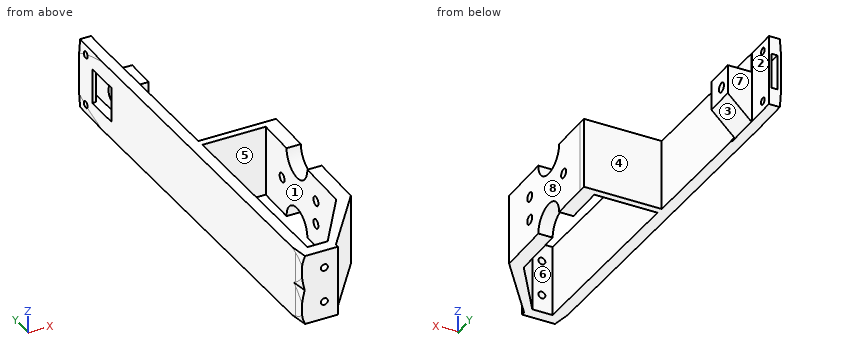
```python
from build123d import *

# Parameters (mm, degrees)
EXTRUDE1_DEPTH                 = 30
EXTRUDE2_DEPTH                 = 30
SKETCH4_R                      = 8.288803623
EXTRUDE4_DEPTH                 = 30
SKETCH5_R                      = 1.95
EXTRUDE5_DEPTH                 = 20
SKETCH6_R                      = 1.95
EXTRUDE6_DEPTH                 = 20
SKETCH9_R                      = 1.45
EXTRUDE9_DEPTH                 = 20
EXTRUDE12_DEPTH                = 171
EXTRUDE15_START                = -4
EXTRUDE15_DEPTH                = 14
SKETCH17_W                     = 15
SKETCH17_H                     = 14.5
EXTRUDE17_DEPTH                = 4
SKETCH18_W                     = 2.5
SKETCH18_H                     = 15
EXTRUDE18_DEPTH                = 10
SKETCH19_W                     = 22
SKETCH19_H                     = 13
EXTRUDE19_DEPTH                = 10
SKETCH20_R                     = 4
EXTRUDE20_DEPTH                = 8.5
SKETCH21_R                     = 2
EXTRUDE21_DEPTH                = 9
EXTRUDE22_DEPTH                = 15
F_2_9_2_9_DIAMETER_HOLE1_D     = 2.9
F_2_9_2_9_DIAMETER_HOLE1_DEPTH = 10
EXTRUDE23_DEPTH                = 32


with BuildPart() as part:
    # Sketch1 → Extrude1 (new body)
    with BuildSketch(Plane.XY):
        Polygon((-0.863115633, -23.253389327), (14.136884367, -23.253389327), (14.136884367, -21.7046417), (34.636884367, 5.336278221), (34.636884367, 61.746610673), (28.636884367, 61.746610673), (28.636884367, 5.55848015), (12.519738096, -18.253389327), (-0.863115633, -18.253389327), align=None)
    extrude(amount=EXTRUDE1_DEPTH)

    # Sketch2 → Extrude2 (add)
    with BuildSketch(Plane.XY):
        Polygon((-0.863115633, -18.253389327), (-4.863115633, 146.746610673), (-0.063115633, 146.746610673), (0.136884367, 146.746610673), (0.136884367, 138.496610673), (1.925187517, 64.729105762), (34.532746461, 64.729105762), (34.636884367, 61.746610673), (28.636884367, 61.746610673), (2.118981118, 61.746610673), (4.058375057, -18.253389327), align=None)
    extrude(amount=EXTRUDE2_DEPTH)

    # Sketch4 → Extrude4 (cut)
    with BuildSketch(Plane(origin=(34.636884367, 0, 0), x_dir=(0, 0, -1), z_dir=(1, 0, 0))):
        with Locations((0, 36.886010892)):
            Circle(SKETCH4_R)
        with Locations((-30, 36.886010892)):
            Circle(SKETCH4_R)
    extrude(amount=-EXTRUDE4_DEPTH, mode=Mode.SUBTRACT)

    # Sketch5 → Extrude5 (cut)
    with BuildSketch(Plane(origin=(34.636884367, 0, 0), x_dir=(0, 0, -1), z_dir=(1, 0, 0))):
        with Locations((-20, 21.746610673)):
            Circle(SKETCH5_R)
        with Locations((-10, 21.746610673)):
            Circle(SKETCH5_R)
    extrude(amount=-EXTRUDE5_DEPTH, mode=Mode.SUBTRACT)

    # Sketch6 → Extrude6 (cut)
    with BuildSketch(Plane(origin=(34.636884367, 0, 0), x_dir=(0, 0, -1), z_dir=(1, 0, 0))):
        with Locations((-15, 48.746610673)):
            Circle(SKETCH6_R)
    extrude(amount=-EXTRUDE6_DEPTH, mode=Mode.SUBTRACT)

    # Sketch9 → Extrude9 (cut)
    with BuildSketch(Plane.XZ.offset(23.253389327)):
        with Locations((8.519738096, 7.5)):
            Circle(SKETCH9_R)
        with Locations((8.519738096, 22.5)):
            Circle(SKETCH9_R)
    extrude(amount=-EXTRUDE9_DEPTH, mode=Mode.SUBTRACT)

    # Sketch14 → Extrude12 (cut, through all)
    with BuildSketch(Plane(origin=(0, 146.746610673, 0), x_dir=(-1, 0, 0), z_dir=(0, 1, 0))):
        with BuildLine():
            Line((4.441840203, 0), (4.863115633, 0))
            Line((4.863115633, 0), (4.863115633, 6.019259174))
            add(Edge.make_bspline(
                [(4.441840203, 0), (4.519153962, 0.855924936), (4.700126089, 2.859430629), (4.803757165, 4.868494671), (4.863115633, 6.019259174)],
                knots=[0, 0, 0, 0, 0.427213628, 1, 1, 1, 1], degree=3))
        make_face()
    extrude12 = extrude(amount=-EXTRUDE12_DEPTH, mode=Mode.SUBTRACT)

    # Sketch15 → Extrude15 (cut)
    with BuildSketch(Plane(origin=(-1.713118599, -23.403267784, 0), x_dir=(-0.984807753, -0.173648178, 0), z_dir=(-0.173648178, 0.984807753, 0)).offset(EXTRUDE15_START)):
        with BuildLine():
            Line((-1.981754914, 15), (2.058740939, 15))
            Line((2.058740939, 15), (2.058740939, 30))
            Line((2.058740939, 30), (-2.130916258, 30))
            add(Edge.make_bspline(
                [(-2.130916258, 30), (-1.660064232, 28.72309887), (-0.852396925, 26.871960577), (-0.491380927, 22.662378444), (-1.504639477, 16.84253988), (-1.773156449, 15.805572323), (-1.981754914, 15)],
                knots=[0, 0, 0, 0, 0.210481429, 0.646187552, 0.725139409, 1, 1, 1, 1], degree=3))
        make_face()
    extrude15 = extrude(amount=EXTRUDE15_DEPTH, mode=Mode.SUBTRACT)

    # Sketch17 → Extrude17 (cut)
    with BuildSketch(Plane(origin=(-1.304855183, -0.031632853, 0), x_dir=(0, 0, 1), z_dir=(-0.999706282, -0.024235304, 0))):
        with Locations((15, 129.571367621)):
            Rectangle(SKETCH17_W, SKETCH17_H)
    extrude(amount=-EXTRUDE17_DEPTH, mode=Mode.SUBTRACT)

    # Sketch18 → Extrude18 (cut)
    with BuildSketch(Plane(origin=(-3.315907411, 136.781180707, 0), x_dir=(0.999706282, 0.024235304, 0), z_dir=(0.024235304, -0.999706282, 0))):
        with Locations((1.444761444, 15)):
            Rectangle(SKETCH18_W, SKETCH18_H)
    extrude(amount=-EXTRUDE18_DEPTH, mode=Mode.SUBTRACT)

    # Sketch19 → Extrude19 (add)
    with BuildSketch(Plane(origin=(0.136884367, 0, 0), x_dir=(0, 0, -1), z_dir=(1, 0, 0))):
        with Locations((-11, 126.496610673)):
            Rectangle(SKETCH19_W, SKETCH19_H)
    extrude(amount=EXTRUDE19_DEPTH)

    # Sketch20 → Extrude20 (cut)
    with BuildSketch(Plane(origin=(2.693969944, 0.065308362, 0), x_dir=(0, 0, 1), z_dir=(-0.999706282, -0.024235304, 0))):
        with Locations((15, 127.621367621)):
            Circle(SKETCH20_R)
    extrude(amount=-EXTRUDE20_DEPTH, mode=Mode.SUBTRACT)

    # Sketch21 → Extrude21 (cut)
    with BuildSketch(Plane(origin=(11.19147334, 0.271308445, 0), x_dir=(0, 0, 1), z_dir=(-0.999706282, -0.024235304, 0))):
        with Locations((15, 127.621367621)):
            Circle(SKETCH21_R)
    extrude(amount=-EXTRUDE21_DEPTH, mode=Mode.SUBTRACT)

    # Sketch22 → Extrude22 (cut)
    with BuildSketch(Plane(origin=(0, 132.996610673, 0), x_dir=(-1, 0, 0), z_dir=(0, 1, 0))):
        Polygon((-0.270217701, 0), (-10.136884367, 9.679287559), (-10.136884367, 0), align=None)
    extrude(amount=-EXTRUDE22_DEPTH, mode=Mode.SUBTRACT)

    # Mirror1: Extrude12 across plane
    add(extrude12.mirror(Plane.XY.offset(15)), mode=Mode.SUBTRACT)

    # Mirror2: Extrude15 across plane
    add(extrude15.mirror(Plane.XY.offset(15)), mode=Mode.SUBTRACT)

    # Ø2.9 (2.9) Diameter Hole1
    with Locations(Plane(origin=(-4.741939114, 141.748079264, 4), x_dir=(0.024235304, -0.999706282, 0), z_dir=(-0.999706282, -0.024235304, 0))):
        with Locations((0, 0)):
            f_2_9_2_9_diameter_hole1 = Hole(F_2_9_2_9_DIAMETER_HOLE1_D / 2, depth=F_2_9_2_9_DIAMETER_HOLE1_DEPTH)

    # Mirror3: Ø2.9 (2.9) Diameter Hole1 across plane
    add(f_2_9_2_9_diameter_hole1.mirror(Plane.XY.offset(15)), mode=Mode.SUBTRACT)

    # Sketch24 → Extrude23 (cut)
    with BuildSketch(Plane.XY.offset(30)):
        Polygon((0.136884367, 138.496610673), (0.136884367, 133.231496822), (0.638228483, 133.231496822), align=None)
    extrude(amount=-EXTRUDE23_DEPTH, mode=Mode.SUBTRACT)


solid = part.part
```
Input: part model. Units: mm. Frame: model coordinates. Face numbers are marked on the shaded views. A direction names the side the tool comes from. Round coordinates to 2 decimals unless told otherwise and drop trailing zeros. Loops run counter-clockwise (first coordinate to the right, second up) from the corner with the lowest first, then second, coordinate; pieces in that order, holes last. Notation, with made-up numbers: (-32.75, 15.5) -> (7.25, 15.5) arc R16 cw to (7.25, 26.5) -> close; hole circle Ø2 at (65, 54.25). An arc over 180 degrees is marked (long way). Use one line per item in the form item = value. Start each with the question number.
Item 1: Mould query, pull axis X, two halves, no side actions, for the marked faces 5, 6, 7 and 8. Classes: pulls with the +X half, pulls with the -X half, needs draft (parallel to the pull), parting line crosses it, or undercut.
Item 2: Contact query for flat-ended pins moving along their axis: pin 1 Ø11 at (y, z) = (141, 10.5) entering from +X; pin 2 Ø11 at (x, y) = (5, 128.5) entering from +Z; pin 3 Ø1.5 at (y, z) = (-20, 19.5) entering from -X; pin 4 Ø6 at (y, z) = (82, 23.5) entering from +X. Output: stop coordinate, or through.
Item 3: Set-up query: the marked faces 1, 2, 3 and 4. Return all of +Z, -Z, +X, -X, +Y, -Y with unobstructed straight access to the full face (end or side cutting, diameter ignored); none if empty.
Item 4: Section query A-A on y = -11. Return the cut outline in (x, z).
Item 5: Material intervals for L1, parallel to Y at x = 32.55, z = 15; L2, parallel to Y at x = 30.85, z = 10; L3, parallel to X at y = 34, z = 8, sorted ascending. Write a range as from..to.
Item 6: Section query C-C on y = 103. Return the cut outline in (x, z), then the cut area to 3 significant figures.
Item 7: Section query B-B on x = 26.5. Return the cut outline in (y, z), then the cut area to 3 significant figures.
Ans:
q1.face_5 = undercut
q1.face_6 = undercut
q1.face_7 = needs draft
q1.face_8 = pulls with the +X half
q2.pin_1 = 0.14
q2.pin_2 = 30
q2.pin_3 = -0.86
q2.pin_4 = 1.58
q3.face_1 = +Z, -Z
q3.face_2 = +Z, -Z, +X, +Y
q3.face_3 = -Z, +X, +Y
q3.face_4 = +Z, -Z, +X
q4.outline = (-1.04, 0) -> (3.88, 0) -> (3.88, 30) -> (-1.04, 30) -> close; (17.43, 0) -> (22.25, 0) -> (22.25, 30) -> (17.43, 30) -> close
q5.L1 = 2.58..46.8, 50.7..64.73
q5.L2 = 0.34..19.8, 23.7..64.73
q5.L3 = -2.13..2.79, 28.64..34.64
q6.outline = (-3.8, 0) -> (1, 0) -> (1, 30) -> (-3.8, 30) -> close
q6.area = 144 mm^2
q7.outline = (-5.4, 0) -> (2.4, 0) -> (2.4, 30) -> (-5.4, 30) -> close; (61.75, 0) -> (64.73, 0) -> (64.73, 30) -> (61.75, 30) -> close
q7.area = 323 mm^2
